Geometry: final body of the model. Coordinates: model frame, mm. A direction names the side the tool comes from. Round coordinates to 2 decimals unless told otherwise and drop trailing zeros. Loops run counter-clockwise (first coordinate to the right, second up) from the corner with the lowest first, then second, coordinate; pieces in that order, holes last. Notation, with made-up numbers: M 85.25,-2 L 124.25,-2 A24 ccw 124.25,26 Z; hole C -19,-16.75 d11. An arc over 180 degrees is marked long. Answer as a JSON object with one key per item and string values.
```python
from build123d import *

# Parameters (mm, degrees)
ESQUISSE1_W             = 150
ESQUISSE1_H             = 240
BASE_EXTRUSION_DEPTH    = 10
ENL_V_MAT_EXTRU_1_DEPTH = 10
ESQUISSE3_R             = 14.142135624
ENL_V_MAT_EXTRU_2_DEPTH = 10


with BuildPart() as part:
    # Esquisse1 → Base-Extrusion (new body)
    with BuildSketch(Plane.XY):
        with Locations((75, 120)):
            Rectangle(ESQUISSE1_W, ESQUISSE1_H)
    extrude(amount=BASE_EXTRUSION_DEPTH)

    # Esquisse2 → Enlèv. mat.-Extru.1 (cut)
    with BuildSketch(Plane.XY.offset(10)):
        with BuildLine():
            Line((53, 0), (97, 0))
            Line((97, 0), (97, 34.679491924))
            ThreePointArc((97, 34.679491924), (75, 80), (53, 34.679491924))
            Line((53, 34.679491924), (53, 0))
        make_face()
    extrude(amount=-ENL_V_MAT_EXTRU_1_DEPTH, mode=Mode.SUBTRACT)

    # Esquisse3 → Enlèv. mat.-Extru.2 (cut)
    with BuildSketch(Plane.XY.offset(10)):
        with Locations((74, 161)):
            Circle(ESQUISSE3_R)
    extrude(amount=-ENL_V_MAT_EXTRU_2_DEPTH, mode=Mode.SUBTRACT)


solid = part.part
```
1) Cut plane C-C on x = 79. Return the cut outline in (y, z).
Geometry results:
{"outline": "M 79.71,0 L 147.77,0 L 147.77,10 L 79.71,10 Z; M 174.23,0 L 240,0 L 240,10 L 174.23,10 Z"}
2) First-contact query: pin 1 (2 mm diameter, centred on x = 58.5, z = 7, fed in from -Y). Flat tip, straight axial feed; report the tip coordinate or a pass-through.
Geometry results:
{"pin 1": "y = 73.86"}
3) Pull-direction query (Y, two-part tool) for faces 3 (the face through (75.877, 79.986, 5.07)), 4 (the face through (74, 122, 10)), 5 (the face through (26, 0, 5)); classes: +Y half, -Y half, draft (parallel to the pull), parting line (faces both ways), or undercut.
Geometry results:
{"face 3": "undercut", "face 4": "draft", "face 5": "-Y half"}
4) Line query: probe 1 along X at (y, z) = (52, 5); probe 2 along Y at (x, z) = (74, 7.75); probe 3 along X at (y, z) = (68.5, 8.25). Output: solid intervals per line, ascending.
Geometry results:
{"probe 1": "0 to 47, 103 to 150", "probe 2": "79.98 to 146.86, 175.14 to 240", "probe 3": "0 to 52.38, 97.62 to 150"}
5) Set-up query: faces 1 (the face through (53, 18, 5)), 2 (the face through (150, 118, 5)). Return all of +Z, -Z, +X, -X, +Y, -Y with unobstructed straight access to the full face (end or side cutting, diameter ignored); none if empty.
Geometry results:
{"face 1": "+Z, -Z, -Y", "face 2": "+Z, -Z, +X, +Y, -Y"}
6) Cut plane B-B on z = 7. Return the cut outline in (x, y), and give its area (3 significant figures).
Geometry results:
{"outline": "M 0,0 L 53,0 L 53,34.68 A28 cw long 97,34.68 L 97,0 L 150,0 L 150,240 L 0,240 Z; hole C 74,161 d28.28", "area": "31,700 mm2"}
7) Cut plane A-A on y = 161. Return the cut outline in (x, z), and give its area (3 significant figures).
Geometry results:
{"outline": "M 0,0 L 59.86,0 L 59.86,10 L 0,10 Z; M 88.14,0 L 150,0 L 150,10 L 88.14,10 Z", "area": "1,220 mm2"}
